CAD build for the part. Positions are in the model's coordinates, mm. A direction names the side the tool comes from. Round coordinates to 2 decimals unless told otherwise and drop trailing zeros. Loops run counter-clockwise (first coordinate to the right, second up) from the corner with the lowest first, then second, coordinate; pieces in that order, holes last.
from build123d import *

# Parameters (mm, degrees)
SKETCH_R        = 1
SKETCH_R_2      = 2
PAD_DEPTH       = 3
POCKET_DEPTH    = 360.627901
POCKET001_DEPTH = 3.001
POCKET002_DEPTH = 360.627901
POCKET005_DEPTH = 3.001


with BuildPart() as part:
    # Sketch → Pad (new body)
    with BuildSketch(Plane.XY):
        with BuildLine():
            Line((-67.5, 28), (47.5, 28))
            Line((87.5, 40), (47.5, 28))
            Line((82.5, -7), (87.5, 40))
            Line((67.5, -7), (82.5, -7))
            Line((67.5, -7), (-67.5, -7))
            ThreePointArc((-67.5, 28), (-85, 10.5), (-67.5, -7))
        make_face()
        with Locations((-50, 4.5)):
            Circle(SKETCH_R, mode=Mode.SUBTRACT)
        with Locations((-50, -4.5)):
            Circle(SKETCH_R, mode=Mode.SUBTRACT)
        with Locations((-50, 0)):
            Circle(SKETCH_R_2, mode=Mode.SUBTRACT)
        with Locations((50, 0)):
            Circle(SKETCH_R_2, mode=Mode.SUBTRACT)
        with Locations((50, 4.5)):
            Circle(SKETCH_R, mode=Mode.SUBTRACT)
        with Locations((50, -4.5)):
            Circle(SKETCH_R, mode=Mode.SUBTRACT)
    extrude(amount=PAD_DEPTH)

    # Sketch001 → Pocket (cut, through all)
    with BuildSketch(Plane.XY.offset(3)):
        with BuildLine():
            Line((-67.5, 11.50065), (-67.5, 8.50065))
            ThreePointArc((-69.002, 8.50065), (-68.251, 7.74965), (-67.5, 8.50065))
            Line((-73.998, 8.50065), (-69.002, 8.50065))
            ThreePointArc((-75.5, 8.50065), (-74.749, 7.74965), (-73.998, 8.50065))
            Line((-75.5, 8.50065), (-75.5, 11.50065))
            ThreePointArc((-73.998, 11.50065), (-74.749, 12.25165), (-75.5, 11.50065))
            Line((-73.998, 11.50065), (-69.002, 11.50065))
            ThreePointArc((-67.5, 11.50065), (-68.251, 12.25165), (-69.002, 11.50065))
        make_face()
        with BuildLine():
            Line((-64.5, 1), (-61.5, 1))
            ThreePointArc((-61.5, -0.502), (-60.749, 0.249), (-61.5, 1))
            Line((-61.5, -0.502), (-61.5, -7))
            Line((-61.5, -7), (-64.5, -7))
            Line((-64.5, -0.502), (-64.5, -7))
            ThreePointArc((-64.5, 1), (-65.251, 0.249), (-64.5, -0.502))
        make_face()
        with BuildLine():
            Line((-64.5, 28), (-61.5, 28))
            Line((-61.5, 21.502), (-61.5, 28))
            ThreePointArc((-61.5, 20), (-60.749, 20.751), (-61.5, 21.502))
            Line((-61.5, 20), (-64.5, 20))
            ThreePointArc((-64.5, 21.502), (-65.251, 20.751), (-64.5, 20))
            Line((-64.5, 28), (-64.5, 21.502))
        make_face()
    pocket = extrude(amount=-POCKET_DEPTH, mode=Mode.SUBTRACT)

    # Mirrored: Pocket across Sketch001 V_Axis
    add(pocket.mirror(Plane(origin=(0, 0, 3), x_dir=(0, 0, 1), z_dir=(1, 0, 0))), mode=Mode.SUBTRACT)

    # Sketch002 → Pocket001 (cut, through all)
    with BuildSketch(Plane.XY.offset(3)):
        with BuildLine():
            ThreePointArc((61.5, 28), (60.749, 27.249), (61.5, 26.498))
            Line((61.5, 26.498), (64.5, 26.498))
            ThreePointArc((64.5, 26.498), (65.251, 27.249), (64.5, 28))
            Line((61.5, 28), (64.5, 28))
        make_face()
    extrude(amount=-POCKET001_DEPTH, mode=Mode.SUBTRACT)

    # Sketch003 → Pocket002 (cut, through all)
    with BuildSketch(Plane.XY.offset(3)):
        with BuildLine():
            Line((-38, -4), (-30, -4))
            ThreePointArc((-30, -5.502), (-29.249, -4.751), (-30, -4))
            Line((-30, -5.502), (-30, -7))
            Line((-30, -7), (-38, -7))
            Line((-38, -5.502), (-38, -7))
            ThreePointArc((-38, -4), (-38.751, -4.751), (-38, -5.502))
        make_face()
    pocket002 = extrude(amount=-POCKET002_DEPTH, mode=Mode.SUBTRACT)

    # Mirrored001: Pocket002 across Sketch003 V_Axis
    add(pocket002.mirror(Plane(origin=(0, 0, 3), x_dir=(0, 0, 1), z_dir=(1, 0, 0))), mode=Mode.SUBTRACT)

    # Sketch008 → Pocket005 (cut, through all)
    with BuildSketch(Plane.XY.offset(3)):
        with BuildLine():
            Line((-48.5, 28), (-56.5, 28))
            Line((-56.5, 28), (-56.5, 26.502))
            ThreePointArc((-56.5, 26.502), (-57.251, 25.751), (-56.5, 25))
            Line((-56.5, 25), (-48.5, 25))
            ThreePointArc((-48.5, 25), (-47.749, 25.751), (-48.5, 26.502))
            Line((-48.5, 28), (-48.5, 26.502))
        make_face()
        with BuildLine():
            Line((77.5, 28), (77.5, 25))
            ThreePointArc((75.998, 25), (76.749, 24.249), (77.5, 25))
            Line((71.002, 25), (75.998, 25))
            ThreePointArc((69.5, 25), (70.251, 24.249), (71.002, 25))
            Line((69.5, 25), (69.5, 28))
            ThreePointArc((71.002, 28), (70.251, 28.751), (69.5, 28))
            Line((71.002, 28), (75.998, 28))
            ThreePointArc((77.5, 28), (76.749, 28.751), (75.998, 28))
        make_face()
    extrude(amount=-POCKET005_DEPTH, mode=Mode.SUBTRACT)


solid = part.part
Item 1: Flat gauge pins, fed straight in: P1, Ø0.9, axis at y = -4.5, z = 1, coming from the -X side; P2, Ø1.5, axis at y = 23.5, z = 1, coming from the -X side; P3, Ø1, axis at x = 15.5, z = 0.5, coming from the +Y side. Where does each tip first touch, or does it go through?
Verdict:
P1: stops at x = -77.22
P2: stops at x = -80
P3: stops at y = 28
Item 2: Wall check: L1, parallel to Y at x = -50, z = 2.3; L2, parallel to Y at x = 50, z = 1.65; L3, parallel to X at y = 5, z = 2.35. Give the ranges that are in metal, low to high.
Verdict:
L1: y = -7 to -5.5, -3.5 to -2, 2 to 3.5, 5.5 to 25
L2: y = -7 to -5.5, -3.5 to -2, 2 to 3.5, 5.5 to 28.75
L3: x = -84.11 to -50.87, -49.13 to 49.13, 50.87 to 83.78
Item 3: 3-axis set-ups, long thin cutter, end or side, ignore diameter. For faces 1 (the flat face through (-75.5, 10, 2)), 2 (the flat face through (34, -4, 2)), 3 (the flat face through (-66, -7, 1)): which of +Z, -Z, +X, -X, +Y, -Y reach the whole face in a straight line?
Verdict:
face 1: +Z, -Z
face 2: +Z, -Z, -Y
face 3: +Z, -Z, +X, -X, -Y
Item 4: Cut at A-A (z = 1.7). State how many separate pieces and enclosed holes the cut face has, plus the area to 3 significant figures.
Verdict:
separate pieces: 1
enclosed holes: 10
area: 5,730 mm2
Item 5: Mould opens along Y. For faces 4 (the flat face through (77.5, 27, 2)), 5 (the flat face through (-61.5, 25, 2)), 6 (the flat face through (50, -7, 1)) say: released by +Y, released by -Y, zero draft, split by the parting line, or undercut.
Verdict:
face 4: undercut
face 5: zero draft
face 6: released by -Y
Item 6: Cut at C-C (y = 17.5). List the corners of the cut face in (x, z), plus the area to 3 significant figures.
Verdict:
outline: (-83.54, 0) - (85.11, 0) - (85.11, 3) - (-83.54, 3) - close
area: 506 mm2
Item 7: Cut at B-B (x = -15). List the corners of the cut face in (y, z).
Verdict:
outline: (-7, 0) - (28, 0) - (28, 3) - (-7, 3) - close
